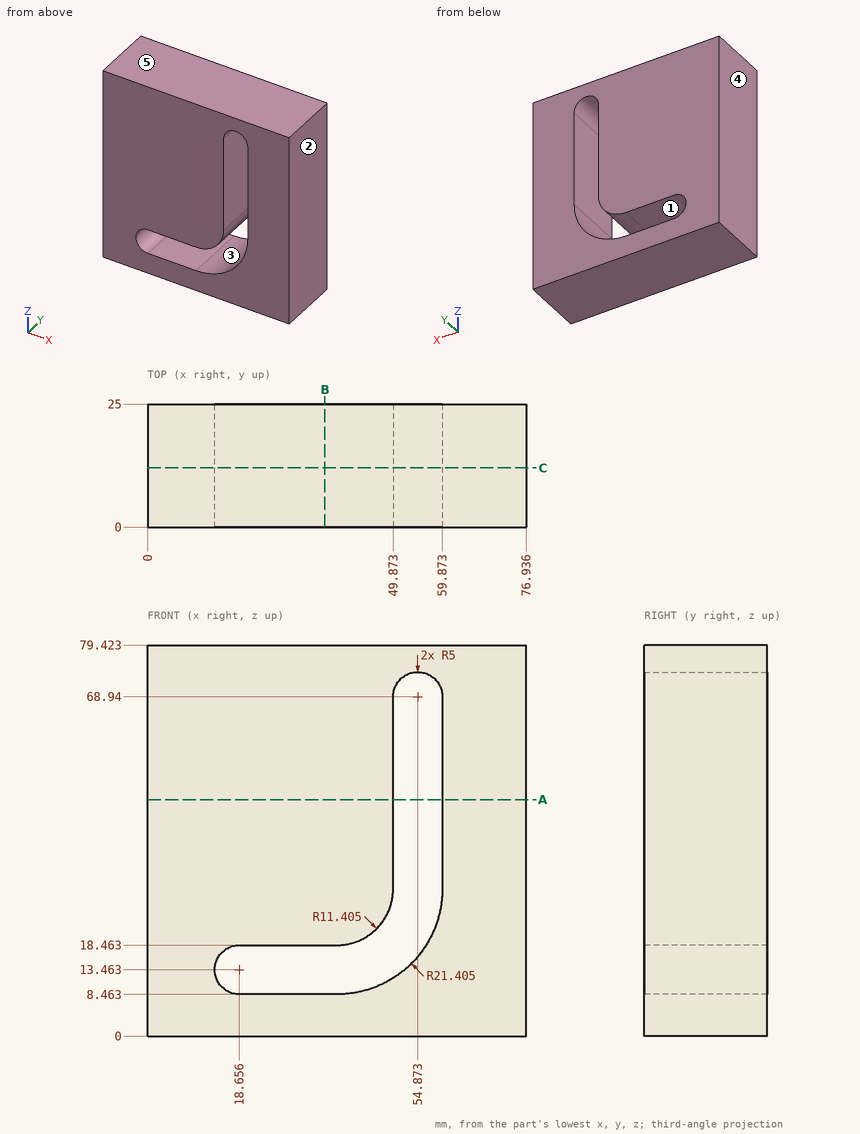
Design review of the part shown in the three views and the two pictorial views. Dimensions are in mm from the part's minimum x, y and z. A direction names the side the tool comes from. Give positions to 0.01 mm unless a question says otherwise; leave off trailing zeros. Write each loop counter-clockwise with the first axis right and the second up, starting at its lowest first coordinate (ties: lowest second). Pieces come first, ordered by that corner, then holes.
Item 1: Wall thickness on probe 1 along Z at (x, y) = (32, 2.5); probe 2 along X at (y, z) = (3.25, 49) (1 decimal); probe 3 along Z at (x, y) = (56, 12.5) (1 decimal): over which ranges is each line inside the solid? List them lowest first.
Item 2: The part is to be moulded in two halves that separate along X. For the marked faces 3, 4 and 5, say which applies: +X half, -X half, draft (parallel to the pull), parting line (faces both ways), or undercut.
Item 3: Take a section at C-C (y = 12). Give the boundary of the cut face in (x, z) (1 decimal).
Item 4: Take a section at A-A (z = 48). Give the boundary of the cut face in (x, y) (1 decimal), and give its area (3 significant figures).
Item 5: Machinability: for the marked faces 1 and 2, which of the approach directions +Z, -Z, +X, -X, +Y, -Y give a long, thin tool a straight path to every point of the face, cutting with its end or side? Answer none if there is none.
Item 6: Take a section at B-B (x = 36). Give the boundary of the cut face in (y, z).
Established:
1. probe 1: z = 0 to 8.46, 18.46 to 79.42
1. probe 2: x = 0 to 49.9, 59.9 to 76.9
1. probe 3: z = 0 to 17.6, 73.8 to 79.4
2. face 3: undercut
2. face 4: -X half
2. face 5: draft
3. outline: (0, 0) - (76.9, 0) - (76.9, 79.4) - (0, 79.4) - close; hole (18.7, 8.5) - (38.5, 8.5) arc R21.4 ccw to (59.9, 29.9) - (59.9, 68.9) arc R5 ccw to (49.9, 68.9) - (49.9, 29.9) arc R11.4 cw to (38.5, 18.5) - (18.7, 18.5) arc R5 ccw to start
4. outline: (0, 0) - (49.9, 0) - (49.9, 25) - (0, 25) - close; (59.9, 0) - (76.9, 0) - (76.9, 25) - (59.9, 25) - close
4. area: 1,670 mm2
5. face 1: +Y, -Y
5. face 2: +Z, -Z, +X, +Y, -Y
6. outline: (0, 0) - (25, 0) - (25, 8.46) - (0, 8.46) - close; (0, 18.46) - (25, 18.46) - (25, 79.42) - (0, 79.42) - close
